```python
from build123d import *

# Parameters (mm, degrees)
PAD_DEPTH = 20
FILLET_R  = 2


with BuildPart() as part:
    # Sketch → Pad (new body)
    with BuildSketch(Plane.XZ):
        Polygon((0, 0), (0, 12), (80, 5), (80, 0), align=None)
    extrude(amount=PAD_DEPTH)

    # Fillet
    fillet_edges = [part.edges().sort_by_distance(p)[0] for p in [
        (0, -10, 0),
        (0, -10, 12),
        (0, 0, 6),
        (0, -20, 6),
        (80, -10, 5),
        (40, 0, 8.5),
        (40, -20, 8.5),
        (80, -10, 0),
        (80, 0, 2.5),
        (80, -20, 2.5),
        (40, 0, 0),
        (40, -20, 0),
    ]]
    fillet(fillet_edges, radius=FILLET_R)


solid = part.part
```
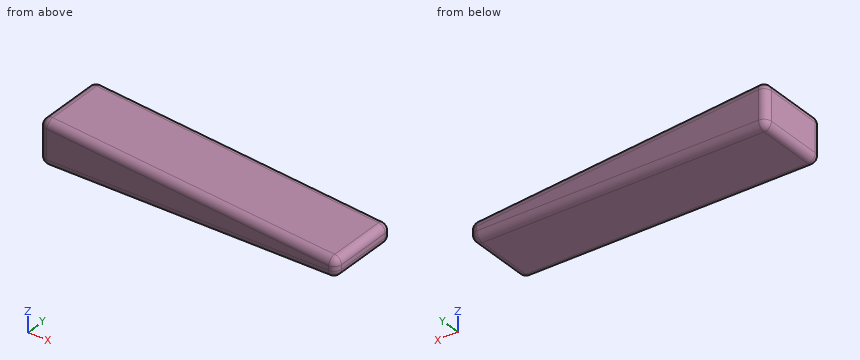
Model file for the job. Use its own axes, mm. Coordinates: 2 decimals unless noted, no trailing zeros. Write each loop counter-clockwise with the first axis right and the second up, starting at its lowest first coordinate (ties: lowest second). Pieces come first, ordered by that corner, then holes. Notation, with made-up numbers: (5, 64) - (11, 64) arc R11 ccw to (11, 75) - close; hole circle Ø9 at (2, 84.5). An arc over 180 degrees is marked (long way). Use a Markdown table: item, result. Add a question column.
Item 1: Band-saw the part on B-B, the plane z = 1. Write the cut outline in (x, y).
Item 2: Drill centre lines: line 1 along X through (y, z) = (-18.25, 2); line 2 along Z through (x, y) = (14, -17.25) (3 decimals); line 3 along Z through (x, y) = (49, -12.75). Where is each one in solid material? Low to high.
Item 3: Drop flat-ended pins along their axis: pin 1 (6 mm diameter, centred on x = 35.5, y = -7.5, fed in from +Z); pin 2 (1.5 mm diameter, centred on x = 43.5, z = 9, fed in from -Y). Give the stop position or say it passes through.
Item 4: Band-saw the part on A-A, the plane y = -9. Write the cut outline in (x, z).
A:
| question | item | result |
|---|---|---|
| 1 | outline | (0.27, -18) arc R1.73 ccw to (2, -19.73) - (78, -19.73) arc R1.73 ccw to (79.73, -18) - (79.73, -2) arc R1.73 ccw to (78, -0.27) - (2, -0.27) arc R1.73 ccw to (0.27, -2) - close |
| 2 | line 1 | x = 0.02 to 79.98 |
| 2 | line 2 | z = 0 to 10.775 |
| 2 | line 3 | z = 0 to 7.71 |
| 3 | pin 1 | stops at z = 9.16 |
| 3 | pin 2 | passes through |
| 4 | outline | (0, 2) arc R2 ccw to (2, 0) - (78, 0) arc R2 ccw to (80, 2) - (80, 3.17) arc R2 ccw to (78.17, 5.16) - (2.17, 11.81) arc R2 ccw to (0, 9.82) - close |
